Here's how the part is built. I have some questions about the finished solid (model axes, mm). Face numbers are marked on the shaded views. A direction names the side the tool comes from. Coordinates: 2 decimals unless noted, no trailing zeros. Order: outer loops, then holes, each group sorted by start corner. A loop starts at its lowest first (then second) coordinate and runs counter-clockwise, first axis right, second up. Notation, with made-up numbers: (71, 51.5) -> (81, 51.5) arc R25 ccw to (81, 69.5) -> close; hole circle Ø9 at (81.5, 89). An arc over 180 degrees is marked (long way). One line per item, written item: value. Start each with the question number.
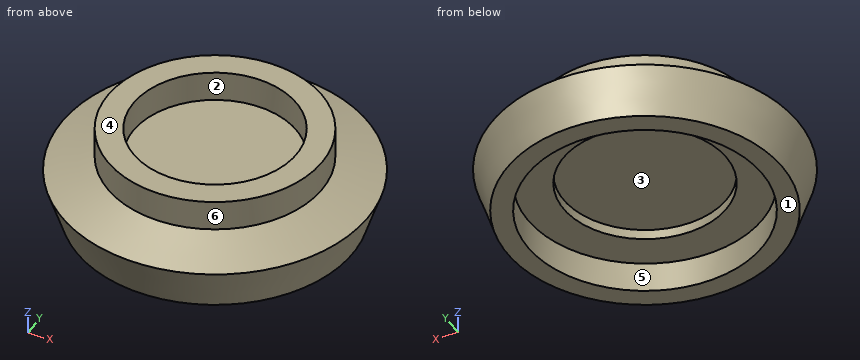
```python
from build123d import *


with BuildPart() as part:
    # Sketch → Revolution (revolve)
    with BuildSketch(Plane.XZ):
        Polygon((-7.5, -0.25), (-5.25, 0.5), (-5.25, 2), (-4, 2), (-4, 0.5), (0, 0.5), (0, -0.5), (-4, -0.5), (-4, -1), (-5.75, -1), (-5.75, -2.5), (-6.75, -2.5), align=None)
    revolve(axis=Axis((0, 0, 0), (0, 0, 1)))


solid = part.part
```
Q1. Imagine slicing it at A-A (y = 0). Write out the boundary of the cut face in (x, z).
Q2. For the marked faces 1, 2 and 3, which set-ups out of +Z, -Z, +X, -X, +Y, -Y let a thin tool reach every point of the face, with its end or its side?
Q3. Imagine slicing it at D-D (z = -1.4). Write out the boundary of the cut face in (x, y).
Q4. I need wall thicknesses on line 1 (X direction, y = 0, z = 1.1); line 2 (Z direction, x = 1.75, y = -4.5). Which ranges of each line are inside material? Lowest first, please.
Q5. Imagine slicing it at C-C (z = 1.65). Write out the boundary of the cut face in (x, y).
Q6. For P1, Ø6.5, axis at x = 0, y = 0, coming from the -Z side; P2, Ø9, axis at x = 0, y = 0, coming from the -Z side; P3, Ø1, axis at x = 5.5, z = -1, coming from the +Y side, each with a flat end and sliding along its axis, tell me the tip position at first contact or that it passes through.
Q7. If we mould it in two halves opening along Y, with no side actions, what happens to the marked faces 4, 5 and 6? For each: +Y half, -Y half, draft (parallel to the pull), parting line (faces both ways), or undercut.
Completed:
1. outline: (-7.5, -0.25) -> (-6.75, -2.5) -> (-5.75, -2.5) -> (-5.75, -1) -> (-4, -1) -> (-4, -0.5) -> (4, -0.5) -> (4, -1) -> (5.75, -1) -> (5.75, -2.5) -> (6.75, -2.5) -> (7.5, -0.25) -> (5.25, 0.5) -> (5.25, 2) -> (4, 2) -> (4, 0.5) -> (-4, 0.5) -> (-4, 2) -> (-5.25, 2) -> (-5.25, 0.5) -> close
2. face 1: -Z, +X, -X, +Y, -Y
2. face 2: +Z
2. face 3: -Z
3. outline: circle Ø14.23 at (0, 0); hole circle Ø11.5 at (0, 0)
4. line 1: x = -5.25 to -4, 4 to 5.25
4. line 2: z = -1 to 2
5. outline: circle Ø10.5 at (0, 0); hole circle Ø8 at (0, 0)
6. P1: stops at z = -0.5
6. P2: stops at z = -1
6. P3: stops at y = 5.3
7. face 4: draft
7. face 5: undercut
7. face 6: parting line
